from build123d import *

# Parameters (mm, degrees)
F0_W     = 19.05
F0_H     = 19.05
F1_DEPTH = 6.35
F2_W     = 12.7
F2_H     = 12.7
F3_DEPTH = 3.74281
F5_DEPTH = 25.4


with BuildPart() as f1:
    # F0 (on Top) → F1 (new body)
    with BuildSketch(Plane.XY):
        Rectangle(F0_W, F0_H)
    extrude(amount=F1_DEPTH)

    # F2 (on face) → F3 (cut)
    with BuildSketch(Plane.XY.offset(6.35)):
        Rectangle(F2_W, F2_H)
    extrude(amount=-F3_DEPTH, mode=Mode.SUBTRACT)

    # F4 (on face) → F5 (cut)
    with BuildSketch(Plane.YZ.offset(9.525)):
        with BuildLine():
            Line((9.525, 6.35), (-9.525, 6.35))
            ThreePointArc((-9.525, 6.35), (0, 4.214056), (9.525, 6.35))
        make_face()
    extrude(amount=-F5_DEPTH, mode=Mode.SUBTRACT)


solid = f1.part
Source: CAD feature listing. Evaluate the final solid. Frame: model axes, mm. A direction names the side the tool comes from. Give positions to 0.01 mm unless a question says otherwise; leave off trailing zeros. Loops run counter-clockwise (first coordinate to the right, second up) from the corner with the lowest first, then second, coordinate; pieces in that order, holes last. Notation, with made-up numbers: (5, 24.25) -> (30, 24.25) arc R11 cw to (30, 45.25) -> close; hole circle Ø2 at (19, 78.25). An arc over 180 degrees is marked (long way). Use a Markdown table: item, result. Add a question column.
1) Line query: line 1 along X through (y, z) = (2.5, 3.25) (3 decimals); line 2 along Z through (x, y) = (2, 6). Output: solid intervals per line, ascending. Write a range as [from, to].
2) Section query A-A, the plane z = 3. Return the cut outline in (x, y) (3 decimals), then the cut area to 3 significant figures.
3) First-contact query: pin 1 (6 mm diameter, centred on x = -6, y = 3.5, fed in from +Z); pin 2 (6.5 mm diameter, centred on x = -1, y = 2, fed in from +Z); pin 3 (1 mm diameter, centred on y = -0.5, z = 5, fed in from +X); pin 4 (10 mm diameter, centred on x = -6, y = -4.5, fed in from +Z). Flat tips, straight axial feed; report the tip coordinate or a pass-through.
4) Section query C-C, the plane y = 0. Return the cut outline in (x, z) (3 decimals).
5) Reachability of faces 5 (the face through (-6.35, 0, 4)), 6 (the face through (0.133, -6.598, 5.212)) from +Z, -Z, +X, -X, +Y, -Y: full face, straight path, thin tool, end or side. Return the list, or none.
6) Pull-direction query (X, two-part tool) for faces 1 (the face through (9.525, 0, 2)), 2 (the face through (-9.525, 0, 2)), 3 (the face through (0, 0, 2.607)), 4 (the face through (0, 0, 0)); classes: +X half, -X half, draft (parallel to the pull), parting line (faces both ways), or undercut.
7) Section query B-B, the plane x = -0.75. Return the cut outline in (y, z) (3 decimals).
8) Section query D-D, the plane x = -7.25. Return the cut outline in (y, z) (3 decimals), then the cut area to 3 significant figures.
Numbers:
| question | item | result |
|---|---|---|
| 1 | line 1 | x = [-9.525, -6.35], [6.35, 9.525] |
| 1 | line 2 | z = [0, 2.61] |
| 2 | outline | (-9.525, -9.525) -> (9.525, -9.525) -> (9.525, 9.525) -> (-9.525, 9.525) -> close; hole (-6.35, -6.35) -> (6.35, -6.35) -> (6.35, 6.35) -> (-6.35, 6.35) -> close |
| 2 | area | 202 mm2 |
| 3 | pin 1 | stops at z = 5.18 |
| 3 | pin 2 | stops at z = 2.61 |
| 3 | pin 3 | passes through |
| 3 | pin 4 | stops at z = 6.34 |
| 4 | outline | (-9.525, 0) -> (9.525, 0) -> (9.525, 4.214) -> (6.35, 4.214) -> (6.35, 2.607) -> (-6.35, 2.607) -> (-6.35, 4.214) -> (-9.525, 4.214) -> close |
| 5 | face 5 | +Z |
| 5 | face 6 | +Z, +X, -X |
| 6 | face 1 | +X half |
| 6 | face 2 | -X half |
| 6 | face 3 | undercut |
| 6 | face 4 | draft |
| 7 | outline | (-9.525, 0) -> (9.525, 0) -> (9.525, 6.35) arc R22.306 cw to (6.35, 5.137) -> (6.35, 2.607) -> (-6.35, 2.607) -> (-6.35, 5.137) arc R22.306 cw to (-9.525, 6.35) -> close |
| 8 | outline | (-9.525, 0) -> (9.525, 0) -> (9.525, 6.35) arc R22.306 cw to (-9.525, 6.35) -> close |
| 8 | area | 93.6 mm2 |
